Read the model definition and answer for the solid it produces. Units are mm, in the model's axes. Face numbers are marked on the shaded views. A direction names the side the tool comes from. Give positions to 0.01 mm unless a question says otherwise; leave off trailing zeros. Order: outer loops, then holes, each group sorted by start corner. A loop starts at its lowest first (then second) coordinate and runs counter-clockwise, first axis right, second up.
Item 1: Find the intervals of material crossed by line 1 along Y through (x, z) = (13, -11.5); line 2 along Z through (x, y) = (1.5, -30); line 3 along Y through (x, z) = (4, 3), in increasing order.
Item 2: A cutting plane is placed at D-D (z = -15). Write down the section's boundary in (x, y).
Item 3: Which of the six approach directions +Z, -Z, +X, -X, +Y, -Y give full straight-line access (tool end or side, diameter ignored) to the marked faces 1, 2, 3 and 4?
Item 4: A cutting plane is placed at C-C (y = -30). Write down the section's boundary in (x, z), plus the area to 3 significant figures.
Item 5: A cutting plane is placed at A-A (x = 0). Write down the section's boundary in (y, z), plus the area to 3 significant figures.
Item 6: Given pin 1 Ø1.5 at (x, z) = (-4.5, 6.5) entering from -Y; pin 2 Ø1 at (x, z) = (13, -14) entering from -Y; pin 3 Ø4 at (x, y) = (8, -10.5) entering from -Z; pin 4 Ø19.5 at (x, z) = (1, -4.5) entering from -Y, each flat-ended and moving along its own axis, determine where each tip first touches the part or whether it passes through.
Item 7: A cutting plane is placed at B-B (z = 9). Write down the section's boundary in (x, y).
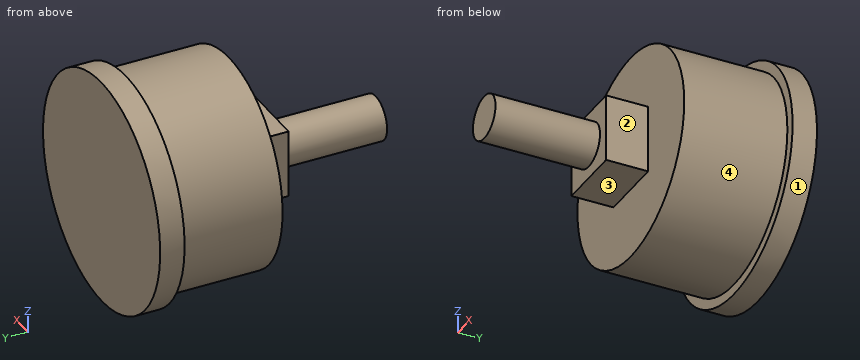
from build123d import *

# Parameters (mm, degrees)
F0_R     = 21.463
F0_R_2   = 19.558
F1_DEPTH = 4.572
F0_W     = 12.7
F0_H     = 12.7
F2_DEPTH = 23.876
F0_R_3   = 4.1275
F3_DEPTH = 31.75
F4_DEPTH = 51.308


with BuildPart() as f1:
    # F0 (on Front) → F1 (new body)
    with BuildSketch(Plane.XZ):
        Circle(F0_R)
        Circle(F0_R_2, mode=Mode.SUBTRACT)
    extrude(amount=F1_DEPTH)

    # F0 (on Front) → F2 (join)
    with BuildSketch(Plane.XZ):
        Circle(F0_R_2)
        Rectangle(F0_W, F0_H, mode=Mode.SUBTRACT)
    extrude(amount=F2_DEPTH)

    # F0 (on Front) → F3 (join)
    with BuildSketch(Plane.XZ):
        Rectangle(F0_W, F0_H)
        Circle(F0_R_3, mode=Mode.SUBTRACT)
    extrude(amount=F3_DEPTH)

    # F0 (on Front) → F4 (join)
    with BuildSketch(Plane.XZ):
        Circle(F0_R_3)
    extrude(amount=F4_DEPTH)


solid = f1.part
Response values:
1. line 1: y = -23.88 to 0
1. line 2: z = -6.35 to 6.35
1. line 3: y = -31.75 to 0
2. outline: (-15.35, -4.57) - (-12.55, -4.57) - (-12.55, -23.88) - (12.55, -23.88) - (12.55, -4.57) - (15.35, -4.57) - (15.35, 0) - (-15.35, 0) - close
3. face 1: +Y, -Y
3. face 2: +Z, -Z, +X, -Y
3. face 3: -Z, +X, -X, -Y
3. face 4: -Y
4. outline: (-6.35, -6.35) - (6.35, -6.35) - (6.35, 6.35) - (-6.35, 6.35) - close
4. area: 161 mm2
5. outline: (-51.31, -4.13) - (-31.75, -4.13) - (-31.75, -6.35) - (-23.88, -6.35) - (-23.88, -19.56) - (-4.57, -19.56) - (-4.57, -21.46) - (0, -21.46) - (0, 21.46) - (-4.57, 21.46) - (-4.57, 19.56) - (-23.88, 19.56) - (-23.88, 6.35) - (-31.75, 6.35) - (-31.75, 4.13) - (-51.31, 4.13) - close
5. area: 1,210 mm2
6. pin 1: stops at y = -31.75
6. pin 2: stops at y = -23.88
6. pin 3: stops at z = -18.61
6. pin 4: stops at y = -51.31
7. outline: (-19.48, -4.57) - (-17.36, -4.57) - (-17.36, -23.88) - (17.36, -23.88) - (17.36, -4.57) - (19.48, -4.57) - (19.48, 0) - (-19.48, 0) - close
